from build123d import *

# Parameters (mm, degrees)
F0_W     = 68.590634
F0_H     = 43.46339
F1_DEPTH = 25.4
F2_D     = 5
F3_R     = 10
F4_DEPTH = 25.401
F5_SIZE  = 5


with BuildPart() as f1:
    # F0 (on Top) → F1 (new body)
    with BuildSketch(Plane.XY):
        Rectangle(F0_W, F0_H)
    extrude(amount=F1_DEPTH)

    # F2 (through all)
    with Locations(Plane(origin=(0, 0, 0), x_dir=(1, 0, 0), z_dir=(0, 0, -1))):
        with Locations((0, 0)):
            Hole(F2_D / 2)

    # F3 (on face) → F4 (cut, through all)
    with BuildSketch(Plane.XY):
        Circle(F3_R)
    extrude(amount=F4_DEPTH, mode=Mode.SUBTRACT)

    # F5
    f5_edges = [f1.edges().sort_by_distance(p)[0] for p in [
        (34.295317, 21.731695, 12.7),
    ]]
    chamfer(f5_edges, length=F5_SIZE)


solid = f1.part
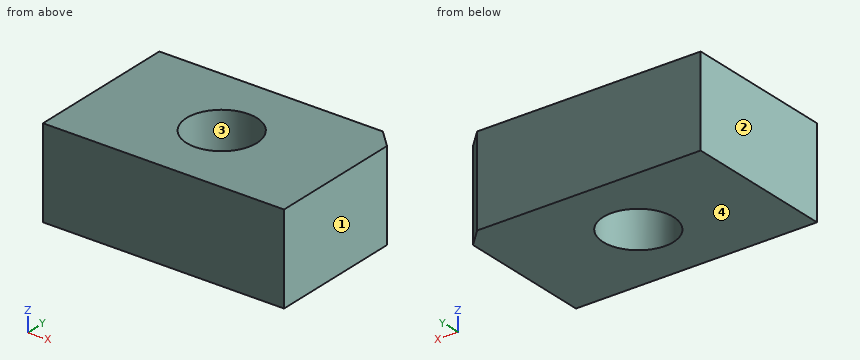
Model file for the job. Use its own axes, mm. Face numbers are marked on the shaded views. Give positions to 0.01 mm unless a question says otherwise; leave off trailing zeros. Loops run counter-clockwise (first coordinate to the right, second up) from the corner with the lowest first, then second, coordinate; pieces in that order, holes last.
1) Flat gauge pin, fed straight in: pin 1 Ø12 at (x, y) = (-17, -2.5) entering from -Z. Where does the tip first touch, or does it go through?
2) Saw through at C-C (z = 14). Write the cut outline in (x, y).
3) Wall check: line 1 (Y direction, x = 0, z = 6); line 2 (X direction, y = 0, z = 15.5); line 3 (X direction, y = 1.5, z = 24). Give the ranges that are in metal, low to high.
4) Saw through at A-A (y = 0). Write the cut outline in (x, z).
5) Pull direction X, two halves, no side cores. Call the marked faces 1, 2, 3 and 4: +X half, -X half, draft (parallel to the pull), parting line (faces both ways), or undercut.
6) Saw through at B-B (x = 0). Write the cut outline in (y, z), plus the area to 3 significant figures.
Answer block:
1. pin 1: stops at z = 0
2. outline: (-34.3, -21.73) - (34.3, -21.73) - (34.3, 16.73) - (29.3, 21.73) - (-34.3, 21.73) - close; hole circle Ø20 at (0, 0)
3. line 1: y = -21.73 to -10, 10 to 21.73
3. line 2: x = -34.3 to -10, 10 to 34.3
3. line 3: x = -34.3 to -9.89, 9.89 to 34.3
4. outline: (-34.3, 0) - (-10, 0) - (-10, 25.4) - (-34.3, 25.4) - close; (10, 0) - (34.3, 0) - (34.3, 25.4) - (10, 25.4) - close
5. face 1: +X half
5. face 2: -X half
5. face 3: undercut
5. face 4: draft
6. outline: (-21.73, 0) - (-10, 0) - (-10, 25.4) - (-21.73, 25.4) - close; (10, 0) - (21.73, 0) - (21.73, 25.4) - (10, 25.4) - close
6. area: 596 mm2
